from build123d import *

# Parameters (mm, degrees)
SKETCH1_R                  = 6.5
SKETCH1_W                  = 19.7
SKETCH1_H                  = 40.64
BASE_FLANGE1_DEPTH         = 1
FILLET1_R                  = 5
F_6_CLEARANCE_HOLE1_D      = 3.7973
SKETCHED_START             = 16.78876
SKETCHED_BEND1_OUTLINE_W   = 115.36
SKETCHED_BEND1_OUTLINE_H   = 1
SKETCHED_BEND1_DEPTH       = 13.21124
SKETCHED_START_2           = -30
SKETCHED_BEND1_2_OUTLINE_W = 115.36
SKETCHED_BEND1_2_OUTLINE_H = 1
SKETCHED_BEND1_2_DEPTH     = 13.18876
SKETCHED_START_3           = -17
SKETCHED_BEND1_3_DEPTH     = 2
SKETCHED_START_4           = 15
SKETCHED_BEND1_4_DEPTH     = 2
SKETCHED_START_5           = -40.18
SKETCHED_BEND1_5_DEPTH     = 115.36
F_4_CLEARANCE_HOLE1_D      = 3.2639
FILLET2_R                  = 1
F_6_CLEARANCE_HOLE2_D      = 3.7973
CUT_EXTRUDE1_DEPTH         = 10


with BuildPart() as part:
    # Base-Flange1: sheet metal written as solids
    # Sketch1 → Base-Flange1 (new body)
    with BuildSketch(Plane.XY):
        Polygon((-30, 75.18), (30, 75.18), (30, -40.18), (15, -40.18), (15, -75.18), (-15, -75.18), (-15, -40.18), (-30, -40.18), align=None)
        with Locations((0, -60.18)):
            Circle(SKETCH1_R, mode=Mode.SUBTRACT)
        Polygon((-26, 60.18), (-19, 54.18), (-19, 36.18), (-26, 30.18), align=None, mode=Mode.SUBTRACT)
        with Locations((0, 45.36)):
            Rectangle(SKETCH1_W, SKETCH1_H, mode=Mode.SUBTRACT)
        Polygon((-26, 24.18), (-19, 30.18), (-19, 0.18), (-26, 6.18), align=None, mode=Mode.SUBTRACT)
        Polygon((-26, -29.82), (-26, 0.18), (-19, -5.82), (-19, -23.82), align=None, mode=Mode.SUBTRACT)
        Polygon((19, -23.82), (26, -29.82), (26, 0.18), (19, -5.82), align=None, mode=Mode.SUBTRACT)
        Polygon((19, 0.18), (26, 6.18), (26, 24.18), (19, 30.18), align=None, mode=Mode.SUBTRACT)
        Polygon((19, 36.18), (26, 30.18), (26, 60.18), (19, 54.18), align=None, mode=Mode.SUBTRACT)
    extrude(amount=-BASE_FLANGE1_DEPTH)

    # Fillet1
    fillet1_edges = [part.edges().sort_by_distance(p)[0] for p in [
        (-30, 75.18, -0.5),
        (30, 75.18, -0.5),
        (30, -40.18, -0.5),
        (15, -75.18, -0.5),
        (-15, -75.18, -0.5),
        (-30, -40.18, -0.5),
    ]]
    fillet(fillet1_edges, radius=FILLET1_R)

    # #6 Clearance Hole1 (through all)
    with Locations(Plane.XY):
        with Locations((-4.97, 70.46), (4.97, 70.46), (-4.97, 20.26), (4.97, 20.26)):
            Hole(F_6_CLEARANCE_HOLE1_D / 2)

    # Sketched Bend1: read off the stored shape, not the designer's step
    # Sketched Bend1 outline → Sketched Bend1 (cut)
    with BuildSketch(Plane.YZ.offset(SKETCHED_START)):
        with Locations((17.5, -0.5)):
            Rectangle(SKETCHED_BEND1_OUTLINE_W, SKETCHED_BEND1_OUTLINE_H)
    extrude(amount=SKETCHED_BEND1_DEPTH, mode=Mode.SUBTRACT)

    # Sketched Bend1 2 outline → Sketched Bend1 2 (cut)
    with BuildSketch(Plane.YZ.offset(SKETCHED_START_2)):
        with Locations((17.5, -0.5)):
            Rectangle(SKETCHED_BEND1_2_OUTLINE_W, SKETCHED_BEND1_2_OUTLINE_H)
    extrude(amount=SKETCHED_BEND1_2_DEPTH, mode=Mode.SUBTRACT)

    # Sketched Bend1 3 outline → Sketched Bend1 3 (add)
    with BuildSketch(Plane.YZ.offset(SKETCHED_START_3)):
        with BuildLine():
            Line((75.18, -9.64380551), (75.18, -1))
            Line((75.18, -1), (-40.18, -1))
            Line((-40.18, -1), (-40.18, -9.64380551))
            ThreePointArc((-40.18, -9.64380551), (-38.715533906, -13.179339416), (-35.18, -14.64380551))
            Line((-35.18, -14.64380551), (70.18, -14.64380551))
            ThreePointArc((70.18, -14.64380551), (73.715533906, -13.179339416), (75.18, -9.64380551))
        make_face()
        Polygon((-23.82, -3.64380551), (-5.82, -3.64380551), (0.18, -10.64380551), (-29.82, -10.64380551), align=None, mode=Mode.SUBTRACT)
        Polygon((0.18, -3.64380551), (30.18, -3.64380551), (24.18, -10.64380551), (6.18, -10.64380551), align=None, mode=Mode.SUBTRACT)
        Polygon((54.18, -3.64380551), (60.18, -10.64380551), (30.18, -10.64380551), (36.18, -3.64380551), align=None, mode=Mode.SUBTRACT)
    extrude(amount=SKETCHED_BEND1_3_DEPTH)

    # Sketched Bend1 4 outline → Sketched Bend1 4 (add)
    with BuildSketch(Plane.YZ.offset(SKETCHED_START_4)):
        with BuildLine():
            Line((75.18, -9.64380551), (75.18, -1))
            Line((75.18, -1), (-40.18, -1))
            Line((-40.18, -1), (-40.18, -9.64380551))
            ThreePointArc((-40.18, -9.64380551), (-38.715533906, -13.179339416), (-35.18, -14.64380551))
            Line((-35.18, -14.64380551), (70.18, -14.64380551))
            ThreePointArc((70.18, -14.64380551), (73.715533906, -13.179339416), (75.18, -9.64380551))
        make_face()
        Polygon((-23.82, -3.64380551), (-5.82, -3.64380551), (0.18, -10.64380551), (-29.82, -10.64380551), align=None, mode=Mode.SUBTRACT)
        Polygon((0.18, -3.64380551), (30.18, -3.64380551), (24.18, -10.64380551), (6.18, -10.64380551), align=None, mode=Mode.SUBTRACT)
        Polygon((54.18, -3.64380551), (60.18, -10.64380551), (30.18, -10.64380551), (36.18, -3.64380551), align=None, mode=Mode.SUBTRACT)
    extrude(amount=SKETCHED_BEND1_4_DEPTH)

    # Sketched Bend1 5 outline → Sketched Bend1 5 (cut)
    with BuildSketch(Plane(origin=(0, 0, 0), x_dir=(1, 0, 0), z_dir=(0, 1, 0)).offset(SKETCHED_START_5)):
        with BuildLine():
            ThreePointArc((-16, 2), (-15.707106781, 1.292893219), (-15, 1))
            Line((-15, 1), (-15, 14.64380551))
            Line((-15, 14.64380551), (-16, 14.64380551))
            Line((-16, 14.64380551), (-16, 2))
        make_face()
        with BuildLine():
            ThreePointArc((17, 2), (16.414213562, 0.585786438), (15, 0))
            Line((15, 0), (16.78876, 0))
            Line((16.78876, 0), (16.78876, 1))
            Line((16.78876, 1), (17, 1))
            Line((17, 1), (17, 2))
        make_face()
        with BuildLine():
            ThreePointArc((-15, 0), (-16.414213562, 0.585786438), (-17, 2))
            Line((-17, 2), (-17, 1))
            Line((-17, 1), (-16.81124, 1))
            Line((-16.81124, 1), (-16.81124, 0))
            Line((-16.81124, 0), (-15, 0))
        make_face()
        with BuildLine():
            ThreePointArc((15, 1), (15.707106781, 1.292893219), (16, 2))
            Line((16, 2), (16, 14.64380551))
            Line((16, 14.64380551), (15, 14.64380551))
            Line((15, 14.64380551), (15, 1))
        make_face()
    extrude(amount=SKETCHED_BEND1_5_DEPTH, mode=Mode.SUBTRACT)

    # #4 Clearance Hole1 (through all)
    with Locations(Plane.XY):
        with Locations((0, -50.18), (0, -70.18)):
            Hole(F_4_CLEARANCE_HOLE1_D / 2)

    # Fillet2
    fillet2_edges = [part.edges().sort_by_distance(p)[0] for p in [
        (-16.5, 54.18, -3.64380551),
        (-16.5, 36.18, -3.64380551),
        (-16.5, 30.18, -10.64380551),
        (-16.5, 60.18, -10.64380551),
        (-16.5, 24.18, -10.64380551),
        (-16.5, 30.18, -3.64380551),
        (-16.5, 0.18, -3.64380551),
        (-16.5, 6.18, -10.64380551),
        (-16.5, -23.82, -3.64380551),
        (-16.5, -29.82, -10.64380551),
        (-16.5, 0.18, -10.64380551),
        (-16.5, -5.82, -3.64380551),
        (16.5, 0.18, -10.64380551),
        (16.5, -29.82, -10.64380551),
        (16.5, -23.82, -3.64380551),
        (16.5, -5.82, -3.64380551),
        (16.5, 24.18, -10.64380551),
        (16.5, 6.18, -10.64380551),
        (16.5, 0.18, -3.64380551),
        (16.5, 30.18, -3.64380551),
        (16.5, 60.18, -10.64380551),
        (16.5, 30.18, -10.64380551),
        (16.5, 36.18, -3.64380551),
        (16.5, 54.18, -3.64380551),
    ]]
    fillet(fillet2_edges, radius=FILLET2_R)

    # #6 Clearance Hole2 (through all)
    with Locations(Plane.XY):
        with Locations((-8, 12), (8, 12), (0, -10.5), (-8, -33), (8, -33)):
            Hole(F_6_CLEARANCE_HOLE2_D / 2)

    # Sketch13 → Cut-Extrude1 (cut)
    with BuildSketch(Plane.XY):
        with BuildLine():
            Line((-7.5, 3), (7.5, 3))
            ThreePointArc((7.5, 3), (10.5, 0), (7.5, -3))
            Line((7.5, -3), (-7.5, -3))
            ThreePointArc((-7.5, -3), (-10.5, 0), (-7.5, 3))
        make_face()
        with BuildLine():
            Line((-7.5, -17), (7.5, -17))
            ThreePointArc((7.5, -17), (10.5, -20), (7.5, -23))
            Line((7.5, -23), (-7.5, -23))
            ThreePointArc((-7.5, -23), (-10.5, -20), (-7.5, -17))
        make_face()
    extrude(amount=-CUT_EXTRUDE1_DEPTH, mode=Mode.SUBTRACT)


solid = part.part
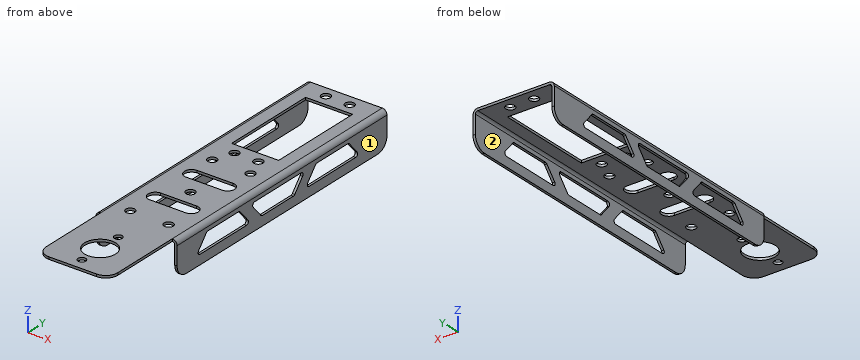
Verification items for the finished model (mm, model axes). Face numbers are marked on the shaded views. A direction names the side the tool comes from. Round coordinates to 2 decimals unless told otherwise and drop trailing zeros. Loops run counter-clockwise (first coordinate to the right, second up) from the corner with the lowest first, then second, coordinate; pieces in that order, holes last. Notation, with made-up numbers: (83.25, 35) - (127.25, 35) arc R14 cw to (127.25, 44) - close; hole circle Ø5 at (67, -4). An arc over 180 degrees is marked (long way). Use a Markdown table: item, result. Add a question column.
1. Section check B-B, the plane x = 0. Give the number of separate pieces and of enclosed holes in the cut face, plus the area to 3 significant figures.
2. Access from +Z, -Z, +X, -X, +Y, -Y to the whole of each face (thin tool, end or side, straight path). Record for the marked faces 1 and 2.
3. Thickness scan on probe 1 along X at (y, z) = (70.46, -0.55); probe 2 along X at (y, z) = (-38.5, -9); probe 3 along Y at (x, z) = (8, -0.2). Record the ranges inside material, lowest first. Write a range as [from, to].
4. Section check A-A, the plane y = 12. Record the boundary of the cut face in (x, z).
5. Section check D-D, the plane y = -57. Record the boundary of the cut face in (x, z), plus the area to 3 significant figures.
6. Gauge pin test, flat ends, axial feed: pin 1 (0.8 mm diameter, centred on x = 16.5, y = 14, fed in from +Z); pin 2 (1 mm diameter, centred on x = -16, z = -4, fed in from -Y); pin 3 (5 mm diameter, centred on y = 6, z = -6, fed in from -X); pin 4 (3 mm diameter, centred on x = 0, y = -50.18, fed in from -Z). Record the tip position at first contact, or that the pin passes through.
Checks:
| question | item | result |
|---|---|---|
| 1 | separate pieces | 8 |
| 1 | enclosed holes | 0 |
| 1 | area | 74.4 mm^2 |
| 2 | face 1 | +Z, -Z, +X, +Y, -Y |
| 2 | face 2 | -Z, +Y, -Y |
| 3 | probe 1 | x = [-16.38, -6.87], [-3.07, 3.07], [6.87, 16.38] |
| 3 | probe 2 | x = [-17, -16], [16, 17] |
| 3 | probe 3 | y = [-75.18, -34.9], [-31.1, -22.96], [-17.04, -2.96], [2.96, 10.1], [13.9, 25.04], [65.68, 75.18] |
| 4 | outline | (-17, -14.64) - (-16, -14.64) - (-16, -10.64) - (-17, -10.64) - close; (-17, -3.64) - (-16, -3.64) - (-16, -2) arc R1 cw to (-15, -1) - (-9.9, -1) - (-9.9, 0) - (-15, 0) arc R2 ccw to (-17, -2) - close; (-6.1, -1) - (6.1, -1) - (6.1, 0) - (-6.1, 0) - close; (9.9, -1) - (15, -1) arc R1 cw to (16, -2) - (16, -3.64) - (17, -3.64) - (17, -2) arc R2 ccw to (15, 0) - (9.9, 0) - close; (16, -14.64) - (17, -14.64) - (17, -10.64) - (16, -10.64) - close |
| 5 | outline | (-15, -1) - (-5.67, -1) - (-5.67, 0) - (-15, 0) - close; (5.67, -1) - (15, -1) - (15, 0) - (5.67, 0) - close |
| 5 | area | 18.7 mm^2 |
| 6 | pin 1 | stops at z = -0.33 |
| 6 | pin 2 | stops at y = -40.18 |
| 6 | pin 3 | stops at x = -17 |
| 6 | pin 4 | passes through |
